from build123d import *

# Parameters (mm, degrees)
SZKIC1_R                    = 21
DODANIE_WYCI_GNI_CIE1_DEPTH = 15
SZKIC6_R                    = 30
DODANIE_WYCI_GNI_CIE3_DEPTH = 5
SZKIC7_R                    = 2.5
WYTNIJ_WYCI_GNI_CIE2_DEPTH  = 5
SZYK_KO_OWY1_COUNT          = 6
SZKIC8_W                    = 37
SZKIC8_H                    = 13
DODANIE_WYCI_GNI_CIE4_DEPTH = 50
SZKIC9_W                    = 36.932370626
SZKIC9_H                    = 10
DODANIE_WYCI_GNI_CIE5_DEPTH = 10
ZAOKR_GLENIE1_R             = 7
ZAOKR_GLENIE2_R             = 7
SZKIC10_R                   = 11
WYTNIJ_WYCI_GNI_CIE3_DEPTH  = 83.800966306
ZAOKR_GLENIE3_R             = 5


# Read off the part's stored shape, not the designer's step: Lustro1
with BuildPart() as part:
    # Szkic1 → Dodanie-wyciągnięcie1 (new body)
    with BuildSketch(Plane.XY):
        Circle(SZKIC1_R)
    extrude(amount=DODANIE_WYCI_GNI_CIE1_DEPTH)

    # Szkic6 → Dodanie-wyciągnięcie3 (add)
    with BuildSketch(Plane.XY.offset(15)):
        Circle(SZKIC6_R)
    extrude(amount=DODANIE_WYCI_GNI_CIE3_DEPTH)

    # Szkic7 → Wytnij-wyciągnięcie2 (cut)
    with BuildSketch(Plane.XY.offset(20)):
        with Locations((0, 25)):
            Circle(SZKIC7_R)
    wytnij_wyci_gni_cie2 = extrude(amount=-WYTNIJ_WYCI_GNI_CIE2_DEPTH, mode=Mode.SUBTRACT)

    # Szyk kołowy1: Wytnij-wyciągnięcie2 ×6 about axis
    szyk_ko_owy1_axis = Axis((0, 0, 0), (0, 0, 1))
    for i in range(1, SZYK_KO_OWY1_COUNT):
        add(wytnij_wyci_gni_cie2.rotate(szyk_ko_owy1_axis, i * 360 / SZYK_KO_OWY1_COUNT), mode=Mode.SUBTRACT)

    # Szkic8 → Dodanie-wyciągnięcie4 (add)
    with BuildSketch(Plane(origin=(0, 0, -40), x_dir=(-1, 0, 0), z_dir=(0, 0, -1))):
        with Locations((0, 26.5)):
            Rectangle(SZKIC8_W, SZKIC8_H)
    extrude(amount=-DODANIE_WYCI_GNI_CIE4_DEPTH)

    # Szkic9 → Dodanie-wyciągnięcie5 (add)
    with BuildSketch(Plane(origin=(0, 10, 0), x_dir=(1, 0, 0), z_dir=(0, 1, 0))):
        with Locations((0, -5)):
            Rectangle(SZKIC9_W, SZKIC9_H)
    extrude(amount=DODANIE_WYCI_GNI_CIE5_DEPTH)

    # Zaokrąglenie1
    # the kernel refuses this fillet: 7 mm, written as the material it adds along each edge
    with BuildSketch(Plane(origin=(-18.466185313, 20, 0), x_dir=(0, 0, -1), z_dir=(1, 0, 0))) as zaokr_glenie1_piece_1:
        with BuildLine():
            CenterArc((ZAOKR_GLENIE1_R, -ZAOKR_GLENIE1_R), ZAOKR_GLENIE1_R, 90, 90)
            Line((0, -ZAOKR_GLENIE1_R), (0, 0))
            Line((0, 0), (ZAOKR_GLENIE1_R, 0))
        make_face()
    extrude(amount=36.932370625)
    with BuildSketch(Plane(origin=(0, 0, 10), x_dir=(0.9435381877974668, -0.33126377430662773, 0), z_dir=(-0.33126377430662773, -0.9435381877974668, 0))) as zaokr_glenie1_piece_2_section:
        with BuildLine():
            CenterArc((21 + ZAOKR_GLENIE1_R, ZAOKR_GLENIE1_R), ZAOKR_GLENIE1_R, 180, 90)
            Line((21 + ZAOKR_GLENIE1_R, 0), (21, 0))
            Line((21, 0), (21, ZAOKR_GLENIE1_R))
        make_face()
    zaokr_glenie1_piece_2 = revolve(axis=Axis((0, 0, 10), (0, 0, 1)), revolution_arc=218.690998802, mode=Mode.PRIVATE)
    zaokr_glenie1_piece_2 = split(zaokr_glenie1_piece_2, bisect_by=Plane(origin=(18.482842321, 20, 10.012675599), z_dir=(0, 1, 0)), keep=Keep.TOP, mode=Mode.PRIVATE)
    zaokr_glenie1_piece_2 = split(zaokr_glenie1_piece_2, bisect_by=Plane(origin=(18.5, 20.258945845, 10.012675599), z_dir=(-1, 0, 0)), keep=Keep.TOP, mode=Mode.PRIVATE)
    zaokr_glenie1_piece_2 = split(zaokr_glenie1_piece_2, bisect_by=Plane(origin=(-18.5, 20.258945845, 10.012675599), z_dir=(1, 0, 0)), keep=Keep.TOP, mode=Mode.PRIVATE)
    add(zaokr_glenie1_piece_2)
    with BuildSketch(Plane(origin=(0, 0, 10), x_dir=(0.9435381877974668, -0.33126377430662773, 0), z_dir=(-0.33126377430662773, -0.9435381877974668, 0))) as zaokr_glenie1_piece_3_section:
        with BuildLine():
            CenterArc((21 + ZAOKR_GLENIE1_R, ZAOKR_GLENIE1_R), ZAOKR_GLENIE1_R, 180, 90)
            Line((21 + ZAOKR_GLENIE1_R, 0), (21, 0))
            Line((21, 0), (21, ZAOKR_GLENIE1_R))
        make_face()
    zaokr_glenie1_piece_3 = revolve(axis=Axis((0, 0, 10), (0, 0, 1)), revolution_arc=218.690998802, mode=Mode.PRIVATE)
    zaokr_glenie1_piece_3 = split(zaokr_glenie1_piece_3, bisect_by=Plane(origin=(18.466185313, 16.543061686, 11.724606468), z_dir=(-1, 0, 0)), keep=Keep.TOP, mode=Mode.PRIVATE)
    zaokr_glenie1_piece_3 = split(zaokr_glenie1_piece_3, bisect_by=Plane(origin=(-18.466185313, 16.543061686, 11.724606468), z_dir=(1, 0, 0)), keep=Keep.TOP, mode=Mode.PRIVATE)
    add(zaokr_glenie1_piece_3)

    # Zaokrąglenie2
    zaokr_glenie2_edges = [part.edges().sort_by_distance(p)[0] for p in [
        (0, 33, 10),
    ]]
    fillet(zaokr_glenie2_edges, radius=ZAOKR_GLENIE2_R)

    # Lustro1: part across plane


with BuildPart() as part_1:
    add(part.part)
    add(part.part.mirror(Plane.ZX))

    # Szkic10 → Wytnij-wyciągnięcie3 (cut, through all)
    with BuildSketch(Plane(origin=(0, 33, 0), x_dir=(1, 0, 0), z_dir=(0, 1, 0))):
        with Locations(Location((0, 20, 0), (0, 0, 180))):
            Circle(SZKIC10_R)
    extrude(amount=-WYTNIJ_WYCI_GNI_CIE3_DEPTH, mode=Mode.SUBTRACT)

    # Zaokrąglenie3
    zaokr_glenie3_edges = [part_1.edges().sort_by_distance(p)[0] for p in [
        (0, -20, -40),
        (18.5, -26.5, -40),
        (0, -33, -40),
        (-18.5, -26.5, -40),
        (0, 33, -40),
        (-18.5, 26.5, -40),
        (18.5, 26.5, -40),
        (0, 20, -40),
    ]]
    fillet(zaokr_glenie3_edges, radius=ZAOKR_GLENIE3_R)


solid = part_1.part
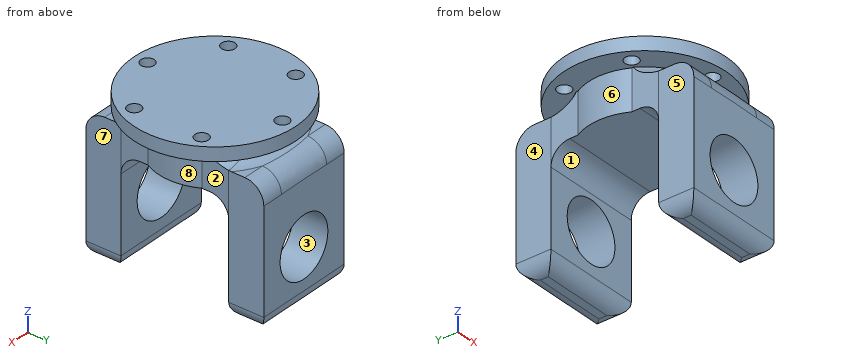
Work out the finished part from the listing and answer in its coordinate system (mm). Face numbers are marked on the shaded views. A direction names the side the tool comes from. Give positions to 0.01 mm unless a question says otherwise; leave off trailing zeros. Order: outer loops, then holes, each group sorted by start corner. A loop starts at its lowest first (then second) coordinate and runs counter-clockwise, first axis right, second up. Notation, with made-up numbers: (50.25, 45.25) -> (84.25, 45.25) arc R12 ccw to (84.25, 49.25) -> close; hole circle Ø7 at (5, 29.25). An arc over 180 degrees is marked (long way). Answer as a JSON object with one key per item and string values. Group by question number.
1. Section B-B on y = 6.5 is taken. Determine the outline of the cut face in (x, z), plus the area to 3 significant figures.
2. Consider line 1 along Y through (x, z) = (0, 17); line 2 along Y through (x, z) = (-15, -33); line 3 along Z through (x, y) = (17.5, -3). Determine where each line is inside the solid, lowest interval first. Write a range as [from, to].
3. A tool of negligible diameter and unlimited length cuts with its end or side. For the marked faces 4, 5, 6, 7 and 8, from which of +Z, -Z, +X, -X, +Y, -Y can it reach the whole face along a straight path? Write none if from no direction.
4. Section A-A on z = -26 is taken. Determine the outline of the cut face in (x, y).
5. Section C-C on x = -1 is taken. Count the separate pieces of the cut face and the enclosed holes in it, plus the area to 3 significant figures.
6. The mould has two halves that part along Z. Classify the marked faces 1, 2 and 3: released by +Z, released by -Z, zero draft, split by the parting line, or undercut.
7. Flat-ended cylindrical pins translate along their axes: pin 1 Ø21 at (x, y) = (6, 3) entering from -Z; pin 2 Ø12 at (x, y) = (14, -12) entering from -Z; pin 3 Ø8 at (y, z) = (17.5, 7.5) entering from +X; pin 4 Ø3 at (x, y) = (-21.65, -12.5) entering from +Z. Find the tip coordinate at first contact, or state that the pin passes through.
8. Section D-D on z = -20 is taken. Determine the outline of the cut face in (x, y).
Result sheet:
{
 "1": {"outline": "(-29.29, 15) -> (-19.97, 15) -> (-19.97, 0) -> (19.97, 0) -> (19.97, 15) -> (29.29, 15) -> (29.29, 20) -> (-29.29, 20) -> close", "area": "892 mm^2"},
 "2": {"line 1": "y = [-30, -27.5], [-22.5, 22.5], [27.5, 30]", "line 2": "y = [-33, -20], [20, 33]", "line 3": "z = [0, 20]"},
 "3": {"face 4": "-Z, -X, +Y", "face 5": "-Z, -X, -Y", "face 6": "-Z, -X", "face 7": "-Z, +X, -Y", "face 8": "-Z, +X"},
 "4": {"outline": "(-18.5, -33) -> (-9.22, -33) -> (-9.22, -20) -> (-18.5, -20) -> close; (-18.5, 20) -> (-9.22, 20) -> (-9.22, 33) -> (-18.5, 33) -> close; (9.22, -33) -> (18.5, -33) -> (18.5, -20) -> (9.22, -20) -> close; (9.22, 20) -> (18.5, 20) -> (18.5, 33) -> (9.22, 33) -> close"},
 "5": {"separate pieces": "5", "enclosed holes": "0", "area": "1,600 mm^2"},
 "6": {"face 1": "released by -Z", "face 2": "zero draft", "face 3": "undercut"},
 "7": {"pin 1": "stops at z = -0.02", "pin 2": "stops at z = -2.1", "pin 3": "stops at x = 18.5", "pin 4": "passes through"},
 "8": {"outline": "(-18.5, -33) -> (-11, -33) -> (-11, -20) -> (-18.5, -20) -> close; (-18.5, 20) -> (-11, 20) -> (-11, 33) -> (-18.5, 33) -> close; (11, -33) -> (18.5, -33) -> (18.5, -20) -> (11, -20) -> close; (11, 20) -> (18.5, 20) -> (18.5, 33) -> (11, 33) -> close"}
}
